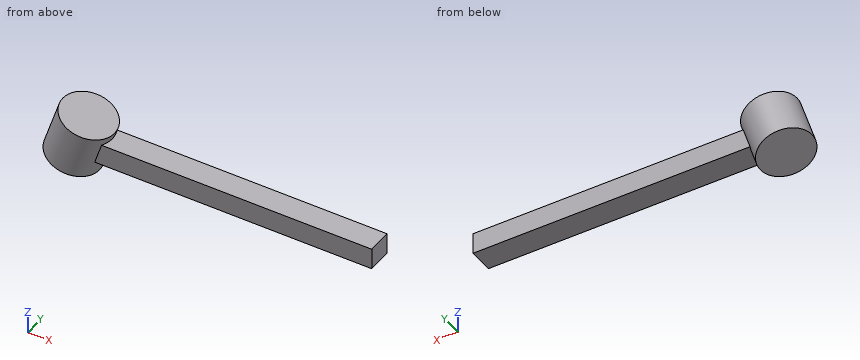
from build123d import *

# Parameters (mm, degrees)
SALIENTE_EXTRUIR1_DEPTH      = 1
SALIENTE_EXTRUIR1_DEPTH_BACK = 1
CROQUIS1_W                   = 25
CROQUIS1_H                   = 1.71875


with BuildPart() as part:
    # Croquis1 → Saliente-Extruir1 (new, two sides: drawn at the far end of the back side and taken through both)
    with BuildSketch(Plane(origin=(0, 0, 0), x_dir=(1, 0, 0), z_dir=(0, 1, 0)).offset(-SALIENTE_EXTRUIR1_DEPTH_BACK)):
        with Locations((5.703125, 0.859375)):
            Rectangle(CROQUIS1_W, CROQUIS1_H)
    extrude(amount=SALIENTE_EXTRUIR1_DEPTH + SALIENTE_EXTRUIR1_DEPTH_BACK)

    # Croquis2 → Revolución1 (revolve)
    with BuildSketch(Plane(origin=(0, 0, 0), x_dir=(1, 0, 0), z_dir=(0, 1, 0))):
        Polygon((-6.49264348, 2.492708525), (-8.58165548, 1.815986328), (-7.37467758, -1.909901974), (-5.285665579, -1.233179777), align=None)
    revolve(axis=Axis((-6.615873756, 0, -2.873115032), (0.3081770108524537, 0, 0.9513290335010526)))


solid = part.part
Geometry: final body of the model. Coordinates: model frame, mm. Round coordinates to 2 decimals unless told otherwise and drop trailing zeros. Loops run counter-clockwise (first coordinate to the right, second up) from the corner with the lowest first, then second, coordinate; pieces in that order, holes last.
Q1. Material intervals for L1, parallel to Z at x = 16, y = -0.6; L2, parallel to Y at x = 1, z = -0.7; L3, parallel to Z at x = -6.5, y = -1.3, sorted ascending.
Q2. Section B-B on y = 0.55. Return loops of the section in (x, z).
Q3. Pin query (flat end, axial travel): P1, Ø1, axis at x = 9.5, y = 0.5, coming from the -Z side; P2, Ø0.6, axis at x = 5, y = 0.5, coming from the +Z side; P3, Ø2, axis at y = 1.5, z = 1.5, coming from the +X side. Return the tip coordinate at first contact, or that it passes through.
Q4. Section A-A on x = -0.5. Return loops of the section in (y, z), plus the area to 3 significant figures.
Q5. Section C-C on y = -1.4. Return loops of the section in (x, z).
Evaluation:
1. L1: z = -1.72 to 0
1. L2: y = -1 to 1
1. L3: z = -2.49 to 1.63
2. outline: (-8.52, -1.84) - (-4.47, -3.15) - (-4.01, -1.72) - (18.2, -1.72) - (18.2, 0) - (-3.45, 0) - (-3.26, 0.58) - (-7.31, 1.89) - close
3. P1: stops at z = -1.72
3. P2: stops at z = 0
3. P3: stops at x = -3.43
4. outline: (-1, -1.72) - (1, -1.72) - (1, 0) - (-1, 0) - close
4. area: 3.44 mm2
5. outline: (-8.1, -1.97) - (-4.88, -3.01) - (-3.68, 0.71) - (-6.9, 1.75) - close
